```python
from build123d import *

# Parameters (mm, degrees)
SKETCH1_R           = 7
BOSS_EXTRUDE1_DEPTH = 2
SKETCH2_R           = 1
BOSS_EXTRUDE2_DEPTH = 2
SKETCH3_R           = 5
BOSS_EXTRUDE3_DEPTH = 20


with BuildPart() as part:
    # Sketch1 → Boss-Extrude1 (new body)
    with BuildSketch(Plane.XY):
        Circle(SKETCH1_R)
    extrude(amount=-BOSS_EXTRUDE1_DEPTH)

    # Sketch2 → Boss-Extrude2 (add)
    with BuildSketch(Plane.XY):
        with Locations((0, 5)):
            Circle(SKETCH2_R)
    extrude(amount=BOSS_EXTRUDE2_DEPTH)

    # Sketch3 → Boss-Extrude3 (add)
    with BuildSketch(Plane(origin=(0, 0, -2), x_dir=(-1, 0, 0), z_dir=(0, 0, -1))):
        Circle(SKETCH3_R)
    extrude(amount=BOSS_EXTRUDE3_DEPTH)


solid = part.part
```
Design review of the part built by this model. Coordinates are the model's own, in mm. A direction names the side the tool comes from. Coordinates: 2 decimals unless noted, no trailing zeros. Write each loop counter-clockwise with the first axis right and the second up, starting at its lowest first coordinate (ties: lowest second). Pieces come first, ordered by that corner, then holes.
1) Add section B-B (x = 2.25). Write out the cut boundary in (y, z).
2) Add section A-A (y = 0). Write out the cut boundary in (x, z).
3) Add section D-D (x = -0.5). Write out the cut boundary in (y, z), plus the area to 3 significant figures.
4) Add section C-C (z = -6.5). Write out the cut boundary in (x, y), plus the area to 3 significant figures.
5) Insertion check: pin 1 (6 mm diameter, centred on x = 3, y = 1.5, fed in from +Z); pin 2 (3 mm diameter, centred on x = 0, z = -19.5, fed in from +Y); pin 3 (1.5 mm diameter, centred on y = -2.5, z = -15, fed in from -X). Each pin has a flat end and moves straight along its axis. Give the tip position at first contact, or say it passes through.
6) Machinability: for faces 1 (the flat face through (0, 0, -22)), 2 (the cylindrical face through (1.08, -4.88, -11.86)), 3 (the cylindrical face through (0, 6, 1)), which of the approach directions +Z, -Z, +X, -X, +Y, -Y give a long, thin tool a straight path to every point of the face, cutting with its end or side? Answer none if there is none.
7) To check wall thickness, follow L1, parallel to Z at x = -2.75, y = 0.25; L2, parallel to X at y = -0.25, z = -4.25; L3, parallel to Z at x = -2, y = 5.5. State the ranges of each line that lie inside material, in increasing order.
Check result:
1. outline: (-6.63, -2) - (-4.47, -2) - (-4.47, -22) - (4.47, -22) - (4.47, -2) - (6.63, -2) - (6.63, 0) - (-6.63, 0) - close
2. outline: (-7, -2) - (-5, -2) - (-5, -22) - (5, -22) - (5, -2) - (7, -2) - (7, 0) - (-7, 0) - close
3. outline: (-6.98, -2) - (-4.97, -2) - (-4.97, -22) - (4.97, -22) - (4.97, -2) - (6.98, -2) - (6.98, 0) - (5.87, 0) - (5.87, 2) - (4.13, 2) - (4.13, 0) - (-6.98, 0) - close
3. area: 230 mm2
4. outline: circle Ø10 at (0, 0)
4. area: 78.5 mm2
5. pin 1: stops at z = 0
5. pin 2: stops at y = 5
5. pin 3: stops at x = -4.68
6. face 1: -Z, +X, -X, +Y, -Y
6. face 2: -Z
6. face 3: +Z
7. L1: z = -22 to 0
7. L2: x = -4.99 to 4.99
7. L3: z = -2 to 0
